from build123d import *

# Parameters (mm, degrees)
SKETCH1_W           = 8
SKETCH1_H           = 20
BOSS_EXTRUDE1_DEPTH = 6
SKETCH2_W           = 4.289164283
SKETCH2_H           = 16.451556892
CUT_EXTRUDE1_DEPTH  = 10
CUT_EXTRUDE2_REACH  = 25.018
SKETCH3_W           = 4.222549804
SKETCH3_H           = 6
SKETCH4_W           = 6
SKETCH4_H           = 4.395289814
BOSS_EXTRUDE2_DEPTH = 3
SKETCH5_W           = 6
SKETCH5_H           = 51.469682585
BOSS_EXTRUDE3_DEPTH = 3
SKETCH6_W           = 6
SKETCH6_H           = 5.271956477
BOSS_EXTRUDE4_DEPTH = 7
SKETCH8_R           = 0.75
CUT_EXTRUDE3_DEPTH  = 56.431741569
SKETCH9_W           = 6
SKETCH9_H           = 4.395289814
BOSS_EXTRUDE5_DEPTH = 3
SKETCH10_R          = 1.15
CUT_EXTRUDE4_DEPTH  = 38.601737593


with BuildPart() as part:
    # Sketch1 → Boss-Extrude1 (new body)
    with BuildSketch(Plane.XY):
        with Locations((-5.686283245, 2.191356499)):
            Rectangle(SKETCH1_W, SKETCH1_H)
    extrude(amount=BOSS_EXTRUDE1_DEPTH)

    # Sketch2 → Cut-Extrude1 (cut)
    with BuildSketch(Plane.XY.offset(6)):
        with Locations((-5.530865387, 1.965578053)):
            Rectangle(SKETCH2_W, SKETCH2_H)
    extrude(amount=-CUT_EXTRUDE1_DEPTH, mode=Mode.SUBTRACT)

    # Sketch3 → Cut-Extrude2 (cut, up to next)
    with BuildSketch(Plane(origin=(0, 12.191356499, 0), x_dir=(1, 0, 0), z_dir=(0, 1, 0)), mode=Mode.PRIVATE) as cut_extrude2_sk1:
        with Locations((-5.525800627, -3)):
            Rectangle(SKETCH3_W, SKETCH3_H)
    cut_extrude2_tool1 = extrude(cut_extrude2_sk1.sketch, amount=-CUT_EXTRUDE2_REACH, mode=Mode.PRIVATE) & part.part
    add(cut_extrude2_tool1.solids().sort_by_distance((-5.525801, 12.191356, 3))[0], mode=Mode.SUBTRACT)

    # Sketch4 → Boss-Extrude2 (add)
    with BuildSketch(Plane(origin=(-1.686283245, 0, 0), x_dir=(0, 0, -1), z_dir=(1, 0, 0))):
        with Locations((-3, 9.993711592)):
            Rectangle(SKETCH4_W, SKETCH4_H)
    extrude(amount=BOSS_EXTRUDE2_DEPTH)

    # Sketch5 → Boss-Extrude3 (add)
    with BuildSketch(Plane.ZY.offset(9.686283245)):
        with Locations((3, 17.926197792)):
            Rectangle(SKETCH5_W, SKETCH5_H)
    extrude(amount=BOSS_EXTRUDE3_DEPTH)

    # Sketch6 → Boss-Extrude4 (add)
    with BuildSketch(Plane.ZY.offset(12.686283245)):
        with Locations((3, 41.025060846)):
            Rectangle(SKETCH6_W, SKETCH6_H)
    extrude(amount=BOSS_EXTRUDE4_DEPTH)

    # Sketch8 → Cut-Extrude3 (cut, through all)
    with BuildSketch(Plane(origin=(0, 43.661039084, 0), x_dir=(1, 0, 0), z_dir=(0, 1, 0))):
        with Locations(Location((-17.186283245, -3, 0), (0, 0, 180))):
            Circle(SKETCH8_R)
    extrude(amount=-CUT_EXTRUDE3_DEPTH, mode=Mode.SUBTRACT)

    # Sketch9 → Boss-Extrude5 (add)
    with BuildSketch(Plane(origin=(1.313716755, 0, 0), x_dir=(0, 0, -1), z_dir=(1, 0, 0))):
        with Locations((-3, 9.993711592)):
            Rectangle(SKETCH9_W, SKETCH9_H)
    extrude(amount=BOSS_EXTRUDE5_DEPTH)

    # Sketch10 → Cut-Extrude4 (cut, through all)
    with BuildSketch(Plane(origin=(0, 12.191356499, 0), x_dir=(1, 0, 0), z_dir=(0, 1, 0))):
        with Locations(Location((1.539504185, -3.336651143, 0), (0, 0, 270))):
            Circle(SKETCH10_R)
    extrude(amount=-CUT_EXTRUDE4_DEPTH, mode=Mode.SUBTRACT)


solid = part.part
Here's how the part is built. I have some questions about the finished solid (model axes, mm). A direction names the side the tool comes from. Coordinates: 2 decimals unless noted, no trailing zeros. Write each loop counter-clockwise with the first axis right and the second up, starting at its lowest first coordinate (ties: lowest second). Pieces come first, ordered by that corner, then holes. Notation, with made-up numbers: (15.5, -29) - (30.5, -29) arc R18 cw to (30.5, -18) - close; hole circle Ø11 at (2.5, 31.5). An arc over 180 degrees is marked (long way). Use one line per item in the form item = value.
1) On a 3-axis mill with a long thin cutter (end or side, diameter ignored), from which of +Z, -Z, +X, -X, +Y, -Y can I reach the whole of each face in a straight line? I mean faces 1 (the flat face through (1, 7.796, 2)), 2 (the flat face through (-7.675, 2, 3)), 3 (the flat face through (-16, 38.389, 3)). Say none if no direction works.
Solved:
face_1 = +Z, -Z, +X, -Y
face_2 = +Z, -Z
face_3 = +Z, -Z, -X, -Y
2) Thinking about a two-plate mould opening in Z: for faces 4 (the flat face through (-7.637, 11, 3)), 5 (the flat face through (-10, 14, 0)), 6 (the cylindrical face through (0.84, 10.024, 2.424)), which applies, released by +Z, released by -Z, zero draft, split by the parting line, or undercut?
Solved:
face_4 = zero draft
face_5 = released by -Z
face_6 = undercut
3) Suppose I cut it at C-C, the plane x = -5.5. Write out the boundary of the cut face in (y, z).
Solved:
outline = (-7.81, 0) - (-6.26, 0) - (-6.26, 6) - (-7.81, 6) - close
4) I need wall thicknesses on line 1 (X direction, y = 6.5, z = 3.5); line 2 (X direction, y = 28, z = 1.65); line 3 (Y direction, x = -12.75, z = 2). Which ranges of each line are inside material? Lowest first, please.
Solved:
line_1 = -12.69 to -7.68, -3.39 to -1.69
line_2 = -12.69 to -9.69
line_3 = 38.39 to 43.66
5) Suppose I cut it at A-A, the plane y = 5. Write out the boundary of the cut face in (x, z).
Solved:
outline = (-12.69, 0) - (-7.68, 0) - (-7.68, 6) - (-12.69, 6) - close; (-3.39, 0) - (-1.69, 0) - (-1.69, 6) - (-3.39, 6) - close
6) I'm going to push flat-ended pins straight in: P1, Ø1.8, axis at x = 1.5, z = 2, coming from the -Y side; P2, Ø3, axis at y = -1.5, z = 4, coming from the -X side; P3, Ø2.5, axis at x = -8, z = 3.5, coming from the +Y side. Where does each tip first touch, or does it pass through?
Solved:
P1 = 7.8
P2 = -12.69
P3 = 12.19
7) Suppose I cut it at B-B, the plane z = 3. Give the number of separate pieces and of enclosed holes in the cut face, plus the area to 3 significant figures.
Solved:
separate_pieces = 3
enclosed_holes = 0
area = 281 mm2
8) Suppose I cut it at D-D, the plane y = 25.5. Write out the boundary of the cut face in (x, z), plus the area to 3 significant figures.
Solved:
outline = (-12.69, 0) - (-9.69, 0) - (-9.69, 6) - (-12.69, 6) - close
area = 18.0 mm2
